from build123d import *

# Parameters (mm, degrees)
SKETCH_1_R               = 4
EXTRUDE_1_DEPTH          = 4
SKETCH_4_R               = 2.5
EXTRUDE_2_DEPTH          = 4
SKETCH_2_R               = 1.6
CUT_EXTRUDE_1_DEPTH      = 4
CUT_EXTRUDE_1_DEPTH_BACK = 3
SKETCH_3_R               = 3.05
CUT_EXTRUDE_2_DEPTH      = 2


with BuildPart() as part:
    # 草图1 → 凸台-拉伸1 (new body)
    with BuildSketch(Plane.XY):
        Circle(SKETCH_1_R)
    extrude(amount=EXTRUDE_1_DEPTH)

    # 草图4 → 凸台-拉伸2 (add)
    with BuildSketch(Plane(origin=(0, 0, 0), x_dir=(-1, 0, 0), z_dir=(0, 0, -1))):
        Circle(SKETCH_4_R)
    extrude(amount=EXTRUDE_2_DEPTH)

    # 草图2 → 切除-拉伸1 (cut, two sides)
    with BuildSketch(Plane(origin=(0, 0, 0), x_dir=(-1, 0, 0), z_dir=(0, 0, -1))) as cut_extrude_1_sk:
        Circle(SKETCH_2_R)
    extrude(amount=CUT_EXTRUDE_1_DEPTH, mode=Mode.SUBTRACT)
    extrude(cut_extrude_1_sk.sketch, amount=-CUT_EXTRUDE_1_DEPTH_BACK, mode=Mode.SUBTRACT)

    # 草图3 → 切除-拉伸2 (cut)
    with BuildSketch(Plane.XY.offset(4)):
        Circle(SKETCH_3_R)
    extrude(amount=-CUT_EXTRUDE_2_DEPTH, mode=Mode.SUBTRACT)


solid = part.part
Part model, mm, in its own coordinate system. A direction names the side the tool comes from. Give positions to 0.01 mm unless a question says otherwise; leave off trailing zeros. Order: outer loops, then holes, each group sorted by start corner. A loop starts at its lowest first (then second) coordinate and runs counter-clockwise, first axis right, second up. Notation, with made-up numbers: (1, -39.75) - (17, -39.75) arc R27 cw to (17, -0.75) - close; hole circle Ø3 at (81.25, 86.25). An arc over 180 degrees is marked (long way). Use a Markdown table: item, result.
1) 3-axis set-ups, long thin cutter, end or side, ignore diameter. For faces 4 (the flat face through (1.3, -1.3, 2)), 5 (the flat face through (0, -2, -4)), 6 (the flat face through (2, 2, 0)): which of +Z, -Z, +X, -X, +Y, -Y reach the whole face in a straight line?
Checked values:
| item | result |
|---|---|
| face 4 | +Z |
| face 5 | -Z, +X, -X, +Y, -Y |
| face 6 | -Z |
2) Saw through at C-C on z = 1.75. List the corners of the cut face in (x, y).
Checked values:
| item | result |
|---|---|
| outline | circle Ø8 at (0, 0); hole circle Ø3.2 at (0, 0) |
3) Two-plate mould, pull along X, no slides. Class faces 1 (the flat face through (0, -3.2, 4)), 2 (the cylindrical face through (-0.867, -3.905, 1.972)), 3 (the cylindrical face through (1.27, -0.97, -0.96)): +X half, -X half, draft (parallel to the pull), parting line (faces both ways), or undercut.
Checked values:
| item | result |
|---|---|
| face 1 | draft |
| face 2 | parting line |
| face 3 | undercut |
4) Saw through at A-A on y = 0. List the corners of the cut face in (x, z).
Checked values:
| item | result |
|---|---|
| outline | (-4, 0) - (-2.5, 0) - (-2.5, -4) - (-1.6, -4) - (-1.6, 2) - (-3.05, 2) - (-3.05, 4) - (-4, 4) - close; (1.6, -4) - (2.5, -4) - (2.5, 0) - (4, 0) - (4, 4) - (3.05, 4) - (3.05, 2) - (1.6, 2) - close |
5) Flat gauge pins, fed straight in: P1, Ø1, axis at x = 3, z = 1.5, coming from the -Y side; P2, Ø1, axis at x = -2.5, z = -3, coming from the +Y side. Where does each tip first touch, or does it go through?
Checked values:
| item | result |
|---|---|
| P1 | y = -3.12 |
| P2 | y = 1.5 |
6) Probe L1, parallel to Y at x = 0, z = -0.05; L2, parallel to Y at x = 0, z = 3.25; L3, parallel to Z at x = -1, y = 1.5. List the from-to ranges inside material, lowest first. Write a range as from..to.
Checked values:
| item | result |
|---|---|
| L1 | -2.5..-1.6, 1.6..2.5 |
| L2 | -4..-3.05, 3.05..4 |
| L3 | -4..2 |
7) Saw through at D-D on x = 2. List the corners of the cut face in (y, z), plus the area to 3 significant figures.
Checked values:
| item | result |
|---|---|
| outline | (-3.46, 0) - (-1.5, 0) - (-1.5, -4) - (1.5, -4) - (1.5, 0) - (3.46, 0) - (3.46, 4) - (2.3, 4) - (2.3, 2) - (-2.3, 2) - (-2.3, 4) - (-3.46, 4) - close |
| area | 30.5 mm² |
